Geometry: final body of the model. Coordinates: model frame, mm. A direction names the side the tool comes from. Coordinates: 2 decimals unless noted, no trailing zeros. Loops run counter-clockwise (first coordinate to the right, second up) from the corner with the lowest first, then second, coordinate; pieces in that order, holes last. Notation, with made-up numbers: M 46,-4 L 70,-4 A13 cw 70,19 Z; hole C 13.5,21 d3. An arc over 180 degrees is marked long. Write each question's results on one line, items separated by ' | '. Start each with the question number.
from build123d import *

# Parameters (mm, degrees)
SKETCH1_W           = 80.01
SKETCH1_H           = 36.068
BOSS_EXTRUDE1_DEPTH = 1.651
SKETCH2_R           = 1.27
CUT_EXTRUDE1_DEPTH  = 2.54
SKETCH3_W           = 71.2978
SKETCH3_H           = 27.1018
BOSS_EXTRUDE2_DEPTH = 8.636
BOSS_EXTRUDE3_DEPTH = 3.1496
SKETCH5_W           = 3.175
SKETCH5_H           = 3.175
BOSS_EXTRUDE4_DEPTH = 2.38125


with BuildPart() as part:
    # Sketch1 → Boss-Extrude1 (new body)
    with BuildSketch(Plane(origin=(0, 0, 0), x_dir=(1, 0, 0), z_dir=(0, 1, 0))):
        with Locations((40.005, 32.202836909)):
            Rectangle(SKETCH1_W, SKETCH1_H)
    extrude(amount=BOSS_EXTRUDE1_DEPTH)

    # Sketch2 → Cut-Extrude1 (cut)
    with BuildSketch(Plane(origin=(0, 1.651, 0), x_dir=(1, 0, 0), z_dir=(0, 1, 0))):
        with Locations(Location((2.54, 47.696836909, 0), (0, 0, 270))):
            Circle(SKETCH2_R)
        with Locations(Location((2.54, 16.708836909, 0), (0, 0, 270))):
            Circle(SKETCH2_R)
        with Locations(Location((77.47, 47.696836909, 0), (0, 0, 270))):
            Circle(SKETCH2_R)
        with Locations(Location((77.47, 16.708836909, 0), (0, 0, 270))):
            Circle(SKETCH2_R)
    extrude(amount=-CUT_EXTRUDE1_DEPTH, mode=Mode.SUBTRACT)

    # Sketch3 → Boss-Extrude2 (add)
    with BuildSketch(Plane(origin=(0, 1.651, 0), x_dir=(1, 0, 0), z_dir=(0, 1, 0))):
        with Locations((40.005, 32.202836909)):
            Rectangle(SKETCH3_W, SKETCH3_H)
    extrude(amount=BOSS_EXTRUDE2_DEPTH)

    # Sketch4 → Boss-Extrude3 (add)
    with BuildSketch(Plane(origin=(0, 1.651, 0), x_dir=(1, 0, 0), z_dir=(0, 1, 0))):
        Polygon((4.3561, 40.203836909), (0, 34.996836909), (0, 29.408836909), (4.3561, 24.201836909), align=None)
    boss_extrude3 = extrude(amount=BOSS_EXTRUDE3_DEPTH)

    # Mirror1: Boss-Extrude3 across plane
    add(boss_extrude3.mirror(Plane.ZY.offset(-40.005)))

    # Sketch5 → Boss-Extrude4 (add)
    with BuildSketch(Plane.XZ):
        with Locations((42.8625, -20.518836909)):
            Rectangle(SKETCH5_W, SKETCH5_H)
    extrude(amount=BOSS_EXTRUDE4_DEPTH)


solid = part.part
Item 1: Section A-A, the plane z = -43.5. Return loops of the section in (x, y), plus the area to 3 significant figures.
Item 2: Contact query for flat-ended pins moving along their axis: P1, Ø2, axis at x = 9, y = 9, coming from the +Z side; P2, Ø5, axis at y = 8, z = -23, coming from the -X side; P3, Ø4, axis at x = 29, z = -26.5, coming from the -Y side. Output: stop coordinate, or through.
Item 3: Section C-C, the plane x = 77.47. Return loops of the section in (y, z), plus the area to 3 significant figures.
Item 4: Section D-D, the plane x = 69. Return loops of the section in (y, z).
Item 5: Set-up query: faces 5 (the flat face through (40, 6, -18.652)), 6 (the flat face through (44.45, -1, -21)), 7 (the flat face through (43, -1, -18.931)). Return all of +Z, -Z, +X, -X, +Y, -Y with unobstructed straight access to the full face (end or side cutting, diameter ignored); none if empty.
Item 6: Ray query, L1, parallel to Z at x = 77.47, y = 0.65; L2, parallel to X at y = 7.5, z = -44; L3, parallel to Y at x = 72.5, z = -22. Return the intervals inside material, ascending. Write a range as [from, to].
Item 7: Section B-B, the plane y = 3.5. Return loops of the section in (x, z), plus the area to 3 significant figures.
Item 8: Pull-direction query (X, two-part tool) for faces 1 (the cylindrical face through (2.054, 0.837, -15.536)), 2 (the flat face through (4.356, 7, -32)), 3 (the flat face through (40, 6, -45.754)), 4 (the cylindrical face through (76.343, 0.837, -16.123)); classes: released by +X, released by -X, zero draft, split by the parting line, or undercut.
Solutions:
1) outline: M 0,0 L 80.01,0 L 80.01,1.65 L 75.65,1.65 L 75.65,10.29 L 4.36,10.29 L 4.36,1.65 L 0,1.65 Z | area: 748 mm²
2) P1: stops at z = -18.65 | P2: stops at x = 4.36 | P3: stops at y = 0
3) outline: M 0,-50.24 L 1.65,-50.24 L 1.65,-48.97 L 0,-48.97 Z; M 0,-46.43 L 1.65,-46.43 L 1.65,-38.03 L 4.8,-38.03 L 4.8,-26.37 L 1.65,-26.37 L 1.65,-17.98 L 0,-17.98 Z; M 0,-15.44 L 1.65,-15.44 L 1.65,-14.17 L 0,-14.17 Z | area: 87.9 mm²
4) outline: M 0,-50.24 L 1.65,-50.24 L 1.65,-45.75 L 10.29,-45.75 L 10.29,-18.65 L 1.65,-18.65 L 1.65,-14.17 L 0,-14.17 Z
5) face 5: +Z, +X, -X, +Y | face 6: +Z, -Z, +X, -Y | face 7: +Z, +X, -X, -Y
6) L1: z = [-50.24, -48.97], [-46.43, -17.98], [-15.44, -14.17] | L2: x = [4.36, 75.65] | L3: y = [0, 10.29]
7) outline: M 0,-35 L 4.36,-40.2 L 4.36,-45.75 L 75.65,-45.75 L 75.65,-40.2 L 80.01,-35 L 80.01,-29.41 L 75.65,-24.2 L 75.65,-18.65 L 4.36,-18.65 L 4.36,-24.2 L 0,-29.41 Z | area: 2,030 mm²
8) face 1: undercut | face 2: released by -X | face 3: zero draft | face 4: undercut
